Geometry check sheet. Reference: the model listing, model coordinates, mm. A direction names the side the tool comes from. Give positions to 0.01 mm unless a question says otherwise; leave off trailing zeros. Write each loop counter-clockwise with the first axis right and the second up, starting at its lowest first coordinate (ties: lowest second). Pieces come first, ordered by that corner, then holes. Notation, with made-up numbers: (42.25, -7.5) -> (92.25, -7.5) arc R23 ccw to (92.25, 16.5) -> close; hole circle Ø8 at (30.5, 68.25). An arc over 180 degrees is marked (long way). One line per item, written item: value.
from build123d import *

# Parameters (mm, degrees)
F0_W           = 50
F0_H           = 80
F1_DEPTH       = 59.182
F2_R           = 8
F4_D           = 17.5
F4_CBORE_D     = 31.5
F4_CBORE_DEPTH = 20
F5_W           = 27.3326538503
F5_H           = 80
F6_DEPTH       = 25
F6_TAPER       = 10
F7_R           = 5


with BuildPart() as f1:
    # F0 (on Top) → F1 (new body)
    with BuildSketch(Plane.XY):
        with Locations((2.3326538503, 22.9340901269)):
            Rectangle(F0_W, F0_H)
    extrude(amount=F1_DEPTH)

    # F2
    f2_edges = [f1.edges().sort_by_distance(p)[0] for p in [
        (-22.667346, 22.93409, 59.182),
        (2.332654, -17.06591, 59.182),
        (27.332654, 22.93409, 59.182),
        (2.332654, 62.93409, 59.182),
    ]]
    fillet(f2_edges, radius=F2_R)

    # F4 (through all)
    with Locations(Plane.XZ.offset(17.0659098731)):
        with Locations((2.3326538503, 24.1386201233)):
            CounterBoreHole(F4_D / 2, F4_CBORE_D / 2, F4_CBORE_DEPTH)

    # F5 (on face) → F6 (join)
    with BuildSketch(Plane(origin=(0, 0, 0), x_dir=(1, 0, 0), z_dir=(0, 0, -1))):
        with Locations((13.6663269252, -22.9340901269)):
            Rectangle(F5_W, F5_H)
    extrude(amount=F6_DEPTH, taper=F6_TAPER)

    # F7
    f7_edges = [f1.edges().sort_by_distance(p)[0] for p in [
        (22.924479, 22.93409, -25),
        (13.666327, -12.657735, -25),
        (4.408175, 22.93409, -25),
        (13.666327, 58.525916, -25),
    ]]
    fillet(f7_edges, radius=F7_R)


solid = f1.part
1) Sectioned sample at C-C on x = -18.5. Record the cut outline in (y, z), plus the area to 3 significant figures.
Verdict:
outline: (-17.07, 0) -> (62.93, 0) -> (62.93, 51.18) arc R8 ccw to (58.77, 58.2) -> (-12.9, 58.2) arc R8 ccw to (-17.07, 51.18) -> close
area: 4,640 mm^2
2) Depth check by flat-ended pin: pin 1 Ø2 at (x, z) = (6.5, -15) entering from -Y; pin 2 Ø2 at (y, z) = (7.5, -6.5) entering from +X; pin 3 Ø7 at (x, y) = (-16.5, 7) entering from -Z. Enter the tip coordinate at first touch or a pass-through.
Verdict:
pin 1: y = -14.6
pin 2: x = 26.36
pin 3: z = 0
3) Sectioned sample at B-B on z = 35.5. Record the cut outline in (x, y), plus the area to 3 significant figures.
Verdict:
outline: (-22.67, -17.07) -> (-8.58, -17.07) -> (-8.58, 2.93) -> (13.24, 2.93) -> (13.24, -17.07) -> (27.33, -17.07) -> (27.33, 62.93) -> (-22.67, 62.93) -> close
area: 3,560 mm^2
4) Scan lines: probe 1 along Z at (x, y) = (10, 47); probe 2 along X at (y, z) = (-11.5, 29); probe 3 along Z at (x, y) = (-4, 43). Record each from-to range of solid material in increasing order.
Verdict:
probe 1: -25 to 19.92, 28.35 to 59.18
probe 2: -22.67 to -12.65, 17.31 to 27.33
probe 3: 0 to 18.1, 30.18 to 59.18
5) Sectioned sample at A-A on x = -10.5. Record the cut outline in (y, z).
Verdict:
outline: (-17.07, 0) -> (62.93, 0) -> (62.93, 51.18) arc R8 ccw to (54.93, 59.18) -> (-9.07, 59.18) arc R8 ccw to (-17.07, 51.18) -> (-17.07, 33.27) -> (2.93, 33.27) -> (2.93, 15.01) -> (-17.07, 15.01) -> close
6) Tool access check on faces 1 (the cylindrical face through (4.229, 33.354, 15.597)), 2 (the cylindrical face through (-10.2, -7.2, 14.6)), 3 (the flat face through (-11, 23, 0)). Record the directions out of +Z, -Z, +X, -X, +Y, -Y that give a thin tool (end or side, any length) a straight path to the whole face; none if there is none.
Verdict:
face 1: +Y, -Y
face 2: -Y
face 3: -Z, -X, +Y, -Y
7) Mould release check, pull along Z, two halves, no side actions. Record for faces 4 (the cylindrical face through (2.68, 60.65, 56.78)), 5 (the flat face through (9, 2.934, 17)), 6 (the flat face through (-22.667, 22, 25)): released by +Z, released by -Z, zero draft, split by the parting line, or undercut.
Verdict:
face 4: released by +Z
face 5: undercut
face 6: zero draft
